from build123d import *

# Parameters (mm, degrees)
SKETCH2_W           = 127
SKETCH2_H           = 76.2
BOSS_EXTRUDE1_DEPTH = 50.8


with BuildPart() as part:
    # Sketch2 → Boss-Extrude1 (new body)
    with BuildSketch(Plane.XY):
        with Locations((63.5, 38.1)):
            Rectangle(SKETCH2_W, SKETCH2_H)
    extrude(amount=BOSS_EXTRUDE1_DEPTH)

    # Sketch5 → CBORE for 1/4 Binding Head Machine Screw1 (revolve, cut)
    with BuildSketch(Plane(origin=(25.4, 25.4, 50.8), x_dir=(0, -1, 0), z_dir=(1, 0, 0))):
        Polygon((0, 0), (0, 50.8), (3.2639, 50.8), (3.2639, 4.191), (7.14375, 4.191), (7.14375, 0.635), (7.77875, 0), align=None)
    revolve(axis=Axis((25.4, 25.4, 57.15), (0, 0, -1)), mode=Mode.SUBTRACT)


solid = part.part
Part model, mm, in its own coordinate system. A direction names the side the tool comes from. Give positions to 0.01 mm unless a question says otherwise; leave off trailing zeros. Order: outer loops, then holes, each group sorted by start corner. A loop starts at its lowest first (then second) coordinate and runs counter-clockwise, first axis right, second up. Notation, with made-up numbers: (78, 31) - (122, 31) arc R11 cw to (122, 37) - close; hole circle Ø8 at (33, 41). An arc over 180 degrees is marked (long way). Use a Markdown table: item, result.
1) Saw through at B-B on x = 25.4. List the corners of the cut face in (y, z) (3 decimals).
Checked values:
| item | result |
|---|---|
| outline | (0, 0) - (22.136, 0) - (22.136, 46.609) - (18.256, 46.609) - (18.256, 50.165) - (17.621, 50.8) - (0, 50.8) - close; (28.664, 0) - (76.2, 0) - (76.2, 50.8) - (33.179, 50.8) - (32.544, 50.165) - (32.544, 46.609) - (28.664, 46.609) - close |
2) Probe L1, parallel to Y at x = 25.4, z = 48.9; L2, parallel to X at y = 25.4, z = 11.5; L3, parallel to Y at x = 25.4, z = 11. List the from-to ranges inside material, lowest first. Write a range as from..to.
Checked values:
| item | result |
|---|---|
| L1 | 0..18.26, 32.54..76.2 |
| L2 | 0..22.14, 28.66..127 |
| L3 | 0..22.14, 28.66..76.2 |
3) Two-plate mould, pull along X, no slides. Class faces 3 (the flat face through (63, 0, 25)), 4 (the flat face through (127, 38, 25)), 5 (the cylindrical face through (22.648, 23.645, 23.631)): +X half, -X half, draft (parallel to the pull), parting line (faces both ways), or undercut.
Checked values:
| item | result |
|---|---|
| face 3 | draft |
| face 4 | +X half |
| face 5 | undercut |
4) Flat gauge pins, fed straight in: P1, Ø2, axis at x = 27.5, z = 12.5, coming from the -Y side; P2, Ø4.5, axis at x = 24, y = 23, coming from the +Z side; P3, Ø5, axis at x = 25.4, y = 25.4, coming from the +Z side. Where does each tip first touch, or does it go through?
Checked values:
| item | result |
|---|---|
| P1 | y = 0 |
| P2 | z = 46.61 |
| P3 | through |
5) 3-axis set-ups, long thin cutter, end or side, ignore diameter. For faces 1 (the flat face through (63, 39, 0)), 2 (the cylindrical face through (20.572, 30.665, 48.412)): which of +Z, -Z, +X, -X, +Y, -Y reach the whole face in a straight line?
Checked values:
| item | result |
|---|---|
| face 1 | -Z, +X, -X, +Y, -Y |
| face 2 | +Z |
6) Saw through at A-A on y = 25.4. List the corners of the cut face in (x, z) (3 decimals).
Checked values:
| item | result |
|---|---|
| outline | (0, 0) - (22.136, 0) - (22.136, 46.609) - (18.256, 46.609) - (18.256, 50.165) - (17.621, 50.8) - (0, 50.8) - close; (28.664, 0) - (127, 0) - (127, 50.8) - (33.179, 50.8) - (32.544, 50.165) - (32.544, 46.609) - (28.664, 46.609) - close |
